from build123d import *

# Parameters (mm, degrees)
ESQUISSE1_W             = 10
ESQUISSE1_H             = 40
BOSS_EXTRU_1_DEPTH      = 300
ENL_V_MAT_EXTRU_1_DEPTH = 303.820078595


with BuildPart() as part:
    # Esquisse1 → Boss.-Extru.1 (new, symmetric)
    with BuildSketch(Plane.XY):
        with Locations((-5, 20)):
            Rectangle(ESQUISSE1_W, ESQUISSE1_H)
    extrude(amount=BOSS_EXTRU_1_DEPTH, both=True)

    # Esquisse2 → Enlèv. mat.-Extru.1 (cut, symmetric)
    with BuildSketch(Plane.XZ):
        Polygon((0, 275), (-10, 285), (-10, 300), (0, 300), align=None)
    enl_v_mat_extru_1 = extrude(amount=ENL_V_MAT_EXTRU_1_DEPTH, both=True, mode=Mode.SUBTRACT)

    # Symétrie1: Enlèv. mat.-Extru.1 across plane
    add(enl_v_mat_extru_1.mirror(Plane.XY), mode=Mode.SUBTRACT)


solid = part.part
Verification items for the finished model (mm, model axes). Give positions to 0.01 mm unless a question says otherwise; leave off trailing zeros. Write each loop counter-clockwise with the first axis right and the second up, starting at its lowest first coordinate (ties: lowest second). Pieces come first, ordered by that corner, then holes.
(1) Cross-section at A-A (x = -2.5). Enter the section's corners in (y, z).
(2) Material ranges on line 1 (Z direction, x = -9, y = 3); line 2 (Z direction, x = -4.5, y = 30.5), recorded low to high.
(3) Cross-section at B-B (y = 5). Enter the section's corners in (x, z).
(4) Gauge pin test, flat ends, axial feed: pin 1 (2 mm diameter, centred on x = -6, y = 26.5, fed in from +Z); pin 2 (2 mm diameter, centred on x = -4.5, y = 8.5, fed in from +Z); pin 3 (4 mm diameter, centred on x = -2.5, y = 24, fed in from +Z). Record the tip position at first contact, or that the pin passes through.
Worked out:
1. outline: (0, -277.5) - (40, -277.5) - (40, 277.5) - (0, 277.5) - close
2. line 1: z = -284 to 284
2. line 2: z = -279.5 to 279.5
3. outline: (-10, -285) - (0, -275) - (0, 275) - (-10, 285) - close
4. pin 1: stops at z = 282
4. pin 2: stops at z = 280.5
4. pin 3: stops at z = 279.5
